Design review of the part built by this model. Coordinates are the model's own, in mm. A direction names the side the tool comes from. Give positions to 0.01 mm unless a question says otherwise; leave off trailing zeros. Write each loop counter-clockwise with the first axis right and the second up, starting at its lowest first coordinate (ties: lowest second). Pieces come first, ordered by that corner, then holes. Notation, with made-up numbers: (75, -31) - (79, -31) arc R13 cw to (79, -13) - close; hole circle Ø3 at (20.25, -18). An arc over 180 degrees is marked (long way). Use a Markdown table: item, result. Add a question column.
```python
from build123d import *

# Parameters (mm, degrees)
F0_W         = 28
F0_H         = 16
F1_DEPTH     = 78
F2_R         = 2.2016502053
F4_DEPTH     = 67.8
F5_R         = 1.5264270503
F6_DEPTH     = 10.6
F3_R         = 8.2210139084
F7_DEPTH     = 5.5
F8_T1_DEPTH  = 68
F8_T3_DEPTH  = 18
F8_T5_DEPTH  = 6
F8_S9_W      = 5
F8_S9_H      = 5
F8_T10_DEPTH = 5
F8_S15_W     = 5
F8_S15_H     = 5
F8_T16_DEPTH = 5
F8_S21_W     = 5
F8_S21_H     = 5
F8_T22_DEPTH = 5
F8_S27_W     = 5
F8_S27_H     = 5
F8_T28_DEPTH = 5
F8_S33_W     = 5
F8_S33_H     = 5
F8_T34_DEPTH = 5
F8_S39_W     = 5
F8_S39_H     = 5
F8_T40_DEPTH = 5
F8_S45_W     = 5
F8_S45_H     = 5
F8_T46_DEPTH = 5
F8_S51_W     = 5
F8_S51_H     = 5
F8_T52_DEPTH = 5


# Not quite as in the source:
# - a fillet or chamfer that OpenCascade refuses, or shapes differently, is made with other operations: its cross-section is extruded or revolved along the edge and cut away or added


with BuildPart() as f1:
    # F0 (on Front) → F1 (new body)
    with BuildSketch(Plane.XZ):
        Rectangle(F0_W, F0_H)
    extrude(amount=F1_DEPTH)

    # F2 (on face) → F4 (cut)
    with BuildSketch(Plane(origin=(0, 0, 0), x_dir=(-1, 0, 0), z_dir=(0, 1, 0))):
        Circle(F2_R)
    extrude(amount=-F4_DEPTH, mode=Mode.SUBTRACT)

    # F5 (on face) → F6 (cut)
    with BuildSketch(Plane(origin=(0, 0, -8), x_dir=(1, 0, 0), z_dir=(0, 0, -1))):
        with Locations((0, 66.9171065092)):
            Circle(F5_R)
    extrude(amount=-F6_DEPTH, mode=Mode.SUBTRACT)

    # F3 (on face) → F7 (cut)
    with BuildSketch(Plane(origin=(0, 0, -8), x_dir=(1, 0, 0), z_dir=(0, 0, -1))):
        with Locations((0, 66.784389317)):
            Circle(F3_R)
    extrude(amount=-F7_DEPTH, mode=Mode.SUBTRACT)

    # F8: fillet of radius 5 on 12 edges, made by hand

    # F8_s2 → F8_t1 (cut)
    with BuildSketch(Plane.XZ.offset(5)):
        with BuildLine():
            ThreePointArc((-14, -3), (-12.5355339059, -6.5355339059), (-9, -8))
            Line((-9, -8), (-14, -8))
            Line((-14, -8), (-14, -3))
        make_face()
        with BuildLine():
            ThreePointArc((14, -3), (12.5355339059, -6.5355339059), (9, -8))
            Line((9, -8), (14, -8))
            Line((14, -8), (14, -3))
        make_face()
        with BuildLine():
            ThreePointArc((9, 8), (12.5355339059, 6.5355339059), (14, 3))
            Line((14, 3), (14, 8))
            Line((14, 8), (9, 8))
        make_face()
        with BuildLine():
            ThreePointArc((-9, 8), (-12.5355339059, 6.5355339059), (-14, 3))
            Line((-14, 3), (-14, 8))
            Line((-14, 8), (-9, 8))
        make_face()
    extrude(amount=F8_T1_DEPTH, mode=Mode.SUBTRACT)

    # F8_s4 → F8_t3 (cut)
    with BuildSketch(Plane.YZ.offset(-9)):
        with BuildLine():
            ThreePointArc((-78, -3), (-76.5355339059, -6.5355339059), (-73, -8))
            Line((-73, -8), (-78, -8))
            Line((-78, -8), (-78, -3))
        make_face()
        with BuildLine():
            ThreePointArc((0, -3), (-1.4644660941, -6.5355339059), (-5, -8))
            Line((-5, -8), (0, -8))
            Line((0, -8), (0, -3))
        make_face()
        with BuildLine():
            ThreePointArc((-5, 8), (-1.4644660941, 6.5355339059), (0, 3))
            Line((0, 3), (0, 8))
            Line((0, 8), (-5, 8))
        make_face()
        with BuildLine():
            ThreePointArc((-73, 8), (-76.5355339059, 6.5355339059), (-78, 3))
            Line((-78, 3), (-78, 8))
            Line((-78, 8), (-73, 8))
        make_face()
    extrude(amount=F8_T3_DEPTH, mode=Mode.SUBTRACT)

    # F8_s6 → F8_t5 (cut)
    with BuildSketch(Plane.XY.offset(-3)):
        with BuildLine():
            ThreePointArc((14, -73), (12.5355339059, -76.5355339059), (9, -78))
            Line((9, -78), (14, -78))
            Line((14, -78), (14, -73))
        make_face()
        with BuildLine():
            ThreePointArc((-14, -73), (-12.5355339059, -76.5355339059), (-9, -78))
            Line((-9, -78), (-14, -78))
            Line((-14, -78), (-14, -73))
        make_face()
        with BuildLine():
            ThreePointArc((-14, -5), (-12.5355339059, -1.4644660941), (-9, 0))
            Line((-9, 0), (-14, 0))
            Line((-14, 0), (-14, -5))
        make_face()
        with BuildLine():
            ThreePointArc((14, -5), (12.5355339059, -1.4644660941), (9, 0))
            Line((9, 0), (14, 0))
            Line((14, 0), (14, -5))
        make_face()
    extrude(amount=F8_T5_DEPTH, mode=Mode.SUBTRACT)


with BuildPart() as f8_tool8:
    # F8_s9 → F8_t10 (new body)
    with BuildSketch(Plane.YZ.offset(-9)):
        with Locations((-2.5, -5.5)):
            Rectangle(F8_S9_W, F8_S9_H)
    extrude(amount=-F8_T10_DEPTH)

    # F8_s11 → F8_t12 (revolve, cut)
    with BuildSketch(Plane(origin=(-9, -5, -3), x_dir=(0, -0.7071067812, 0.7071067812), z_dir=(0, -0.7071067812, -0.7071067812))):
        with BuildLine():
            ThreePointArc((0, -5), (5, 0), (0, 5))
            Line((0, 5), (0, -5))
        make_face()
    revolve(axis=Axis((-9, -5, -3), (-1, 0, 0)), mode=Mode.SUBTRACT)


with BuildPart() as f1_1:
    add(f1.part)

    # F8_t7: cut F8_tool8
    add(f8_tool8.part, mode=Mode.SUBTRACT)


with BuildPart() as f8_tool14:
    # F8_s15 → F8_t16 (new body)
    with BuildSketch(Plane.YZ.offset(-9)):
        with Locations((-75.5, -5.5)):
            Rectangle(F8_S15_W, F8_S15_H)
    extrude(amount=-F8_T16_DEPTH)

    # F8_s17 → F8_t18 (revolve, cut)
    with BuildSketch(Plane(origin=(-9, -73, -3), x_dir=(0, 0.7071067812, 0.7071067812), z_dir=(0, -0.7071067812, 0.7071067812))):
        with BuildLine():
            ThreePointArc((0, -5), (5, 0), (0, 5))
            Line((0, 5), (0, -5))
        make_face()
    revolve(axis=Axis((-9, -73, -3), (-1, 0, 0)), mode=Mode.SUBTRACT)


with BuildPart() as f1_2:
    add(f1_1.part)

    # F8_t13: cut F8_tool14
    add(f8_tool14.part, mode=Mode.SUBTRACT)


with BuildPart() as f8_tool20:
    # F8_s21 → F8_t22 (new body)
    with BuildSketch(Plane.YZ.offset(9)):
        with Locations((-75.5, -5.5)):
            Rectangle(F8_S21_W, F8_S21_H)
    extrude(amount=F8_T22_DEPTH)

    # F8_s23 → F8_t24 (revolve, cut)
    with BuildSketch(Plane(origin=(9, -73, -3), x_dir=(0, 0.7071067812, 0.7071067812), z_dir=(0, 0.7071067812, -0.7071067812))):
        with BuildLine():
            ThreePointArc((0, -5), (5, 0), (0, 5))
            Line((0, 5), (0, -5))
        make_face()
    revolve(axis=Axis((9, -73, -3), (1, 0, 0)), mode=Mode.SUBTRACT)


with BuildPart() as f1_3:
    add(f1_2.part)

    # F8_t19: cut F8_tool20
    add(f8_tool20.part, mode=Mode.SUBTRACT)


with BuildPart() as f8_tool26:
    # F8_s27 → F8_t28 (new body)
    with BuildSketch(Plane.YZ.offset(9)):
        with Locations((-2.5, -5.5)):
            Rectangle(F8_S27_W, F8_S27_H)
    extrude(amount=F8_T28_DEPTH)

    # F8_s29 → F8_t30 (revolve, cut)
    with BuildSketch(Plane(origin=(9, -5, -3), x_dir=(0, -0.7071067812, 0.7071067812), z_dir=(0, 0.7071067812, 0.7071067812))):
        with BuildLine():
            ThreePointArc((0, -5), (5, 0), (0, 5))
            Line((0, 5), (0, -5))
        make_face()
    revolve(axis=Axis((9, -5, -3), (1, 0, 0)), mode=Mode.SUBTRACT)


with BuildPart() as f1_4:
    add(f1_3.part)

    # F8_t25: cut F8_tool26
    add(f8_tool26.part, mode=Mode.SUBTRACT)


with BuildPart() as f8_tool32:
    # F8_s33 → F8_t34 (new body)
    with BuildSketch(Plane.XY.offset(3)):
        with Locations((11.5, -2.5)):
            Rectangle(F8_S33_W, F8_S33_H)
    extrude(amount=F8_T34_DEPTH)

    # F8_s35 → F8_t36 (revolve, cut)
    with BuildSketch(Plane(origin=(9, -5, 3), x_dir=(-0.7071067812, -0.7071067812, 0), z_dir=(-0.7071067812, 0.7071067812, 0))):
        with BuildLine():
            ThreePointArc((0, -5), (5, 0), (0, 5))
            Line((0, 5), (0, -5))
        make_face()
    revolve(axis=Axis((9, -5, 3), (0, 0, 1)), mode=Mode.SUBTRACT)


with BuildPart() as f1_5:
    add(f1_4.part)

    # F8_t31: cut F8_tool32
    add(f8_tool32.part, mode=Mode.SUBTRACT)


with BuildPart() as f8_tool38:
    # F8_s39 → F8_t40 (new body)
    with BuildSketch(Plane.XY.offset(3)):
        with Locations((-11.5, -2.5)):
            Rectangle(F8_S39_W, F8_S39_H)
    extrude(amount=F8_T40_DEPTH)

    # F8_s41 → F8_t42 (revolve, cut)
    with BuildSketch(Plane(origin=(-9, -5, 3), x_dir=(0.7071067812, -0.7071067812, 0), z_dir=(-0.7071067812, -0.7071067812, 0))):
        with BuildLine():
            ThreePointArc((0, -5), (5, 0), (0, 5))
            Line((0, 5), (0, -5))
        make_face()
    revolve(axis=Axis((-9, -5, 3), (0, 0, 1)), mode=Mode.SUBTRACT)


with BuildPart() as f1_6:
    add(f1_5.part)

    # F8_t37: cut F8_tool38
    add(f8_tool38.part, mode=Mode.SUBTRACT)


with BuildPart() as f8_tool44:
    # F8_s45 → F8_t46 (new body)
    with BuildSketch(Plane.XY.offset(3)):
        with Locations((11.5, -75.5)):
            Rectangle(F8_S45_W, F8_S45_H)
    extrude(amount=F8_T46_DEPTH)

    # F8_s47 → F8_t48 (revolve, cut)
    with BuildSketch(Plane(origin=(9, -73, 3), x_dir=(-0.7071067812, 0.7071067812, 0), z_dir=(0.7071067812, 0.7071067812, 0))):
        with BuildLine():
            ThreePointArc((0, -5), (5, 0), (0, 5))
            Line((0, 5), (0, -5))
        make_face()
    revolve(axis=Axis((9, -73, 3), (0, 0, 1)), mode=Mode.SUBTRACT)


with BuildPart() as f1_7:
    add(f1_6.part)

    # F8_t43: cut F8_tool44
    add(f8_tool44.part, mode=Mode.SUBTRACT)


with BuildPart() as f8_tool50:
    # F8_s51 → F8_t52 (new body)
    with BuildSketch(Plane.XY.offset(3)):
        with Locations((-11.5, -75.5)):
            Rectangle(F8_S51_W, F8_S51_H)
    extrude(amount=F8_T52_DEPTH)

    # F8_s53 → F8_t54 (revolve, cut)
    with BuildSketch(Plane(origin=(-9, -73, 3), x_dir=(0.7071067812, 0.7071067812, 0), z_dir=(0.7071067812, -0.7071067812, 0))):
        with BuildLine():
            ThreePointArc((0, -5), (5, 0), (0, 5))
            Line((0, 5), (0, -5))
        make_face()
    revolve(axis=Axis((-9, -73, 3), (0, 0, 1)), mode=Mode.SUBTRACT)


with BuildPart() as f1_8:
    add(f1_7.part)

    # F8_t49: cut F8_tool50
    add(f8_tool50.part, mode=Mode.SUBTRACT)


solid = f1_8.part
```
(1) Add section B-B (x = 0). State the section outline as (y, z) points.
(2) Add section C-C (z = 0). State the section outline as (x, y) points.
(3) Mouldability with a two-part tool opening along Y and no side actions: class faces 1 (the face through (-13, -39, -6)), 2 (the face through (-1.78, -58.76, -5.29)), 3 (the face through (0, -77, -6)), 4 (the face through (0, -2, 7)) as +Y half, -Y half, draft (parallel to the pull), parting line (faces both ways), or undercut.
(4) For line 1 along X through (y, z) = (-44, 0); line 2 along Z through (x, y) = (-6.75, -68); line 3 along Y through (x, z) = (3.5, -4.25), list the stretches that pass through material, from the lowest coordinate up.
(5) Tool access review of faces 5 (the face through (12, -39, 7)), 6 (the face through (-2.1, -33.43, 0.66)), 7 (the face through (0, -65, -2.5)): name each direction out of +Z, -Z, +X, -X, +Y, -Y from which nothing blocks a thin tool from reaching the whole face with its end or side.
(6) Insertion check: pin 1 (0.9 mm diameter, centred on x = 0, y = -67, fed in from -Z); pin 2 (3.5 mm diameter, centred on x = 0, z = 0, fed in from +Y); pin 3 (3 mm diameter, centred on y = -47.5, z = -6, fed in from +X). Each pin has a flat end and moves straight along its axis. Give the tip position at first contact, or say it passes through.
(7) Add section A-A (y = -39.5). State the section outline as (x, z) points.
(8) Add section D-D (x = -12). State the section outline as (y, z) points.
Answers follow:
| question | item | result |
|---|---|---|
| 1 | outline | (-78, -3) arc R5 ccw to (-75.01, -7.58) - (-75.01, -2.5) - (-68.44, -2.5) - (-68.44, 2.6) - (-65.39, 2.6) - (-65.39, 2.2) - (0, 2.2) - (0, 3) arc R5 ccw to (-5, 8) - (-73, 8) arc R5 ccw to (-78, 3) - close; (-65.39, -2.5) - (-58.56, -2.5) - (-58.56, -8) - (-5, -8) arc R5 ccw to (0, -3) - (0, -2.2) - (-65.39, -2.2) - close |
| 2 | outline | (-14, -73) arc R5 ccw to (-9, -78) - (9, -78) arc R5 ccw to (14, -73) - (14, -5) arc R5 ccw to (9, 0) - (2.2, 0) - (2.2, -67.8) - (1.25, -67.8) arc R1.53 cw to (-1.25, -67.8) - (-2.2, -67.8) - (-2.2, 0) - (-9, 0) arc R5 ccw to (-14, -5) - close |
| 3 | face 1 | draft |
| 3 | face 2 | undercut |
| 3 | face 3 | -Y half |
| 3 | face 4 | +Y half |
| 4 | line 1 | -14 to -2.2, 2.2 to 14 |
| 4 | line 2 | -2.5 to 8 |
| 4 | line 3 | -77.84 to -74.22, -59.35 to -0.16 |
| 5 | face 5 | +Z, +X, +Y, -Y |
| 5 | face 6 | +Y |
| 5 | face 7 | -Z |
| 6 | pin 1 | z = 2.6 |
| 6 | pin 2 | y = -67.8 |
| 6 | pin 3 | x = 13.77 |
| 7 | outline | (-14, -3) arc R5 ccw to (-9, -8) - (9, -8) arc R5 ccw to (14, -3) - (14, 3) arc R5 ccw to (9, 8) - (-9, 8) arc R5 ccw to (-14, 3) - close; hole circle Ø4.4 at (0, 0) |
| 8 | outline | (-77, -3) arc R4 ccw to (-73, -7) - (-5, -7) arc R4 ccw to (-1, -3) - (-1, 3) arc R4 ccw to (-5, 7) - (-73, 7) arc R4 ccw to (-77, 3) - close |
